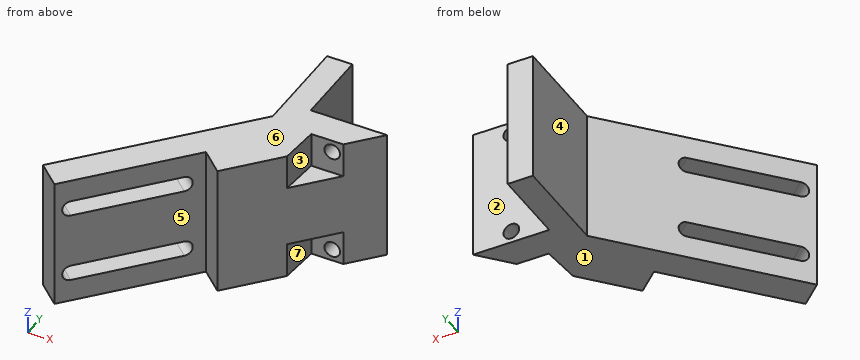
Autodesk Inventor part; units mm, degrees
ref_plane "Work Plane2" through (-4.445, -9.144, -33.02) normal (0, 0, -1) x (0, 1, 0)
ref_plane "YZ Plane" through (0, 0, 0) normal (1, 0, 0) x (0, 1, 0)
ref_plane "XZ Plane" through (0, 0, 0) normal (0, 1, 0) x (-1, 0, 0)
ref_plane "Work Plane1" through (0, 0, 0) normal (0, 0, 1) x (1, 0, 0)
sketch "Sketch1" plane through (0, 0, 0) normal (0, 0, 1) x (1, 0, 0)
  line L0 (4.129202, -9.5377) -> (6.406797, -9.5377) construction
  line L1 (9.525, -8.41296) -> (9.525, -7.435497) construction
  line L2 (-6.406797, 9.5123) -> (-4.129202, 9.5123) construction
  line L3 (-9.525, 4.116502) -> (-9.525, 6.394097) construction
  line L4 (9.314549, -9.373063) -> (-73.965447, -101.864868) construction
  line L5 (9.166309, -9.5377) -> (-73.965447, -101.864868)
  line L6 (-73.965447, -101.864868) -> (-85.121243, -91.820144)
  line L7 (6.33881, 9.756536) -> (-85.121243, -91.820144) construction
  line L8 (9.166309, -9.5377) -> (-9.997679, -9.5377)
  line L9 (-9.997679, -9.5377) -> (-9.997679, 9.756536)
  line L10 (-9.997679, 9.756536) -> (-16.347679, 9.756536)
  line L11 (-16.347679, 9.756536) -> (-16.347679, -15.439362)
  line L12 (-16.347679, -15.439362) -> (-85.121243, -91.820144)
  point P0 (0, 0)
  dimension "d0" = 124.46
  dimension "d1" = 48
  dimension "d5" = 6.35
ref_plane "Work Plane2" through (-4.445, -9.144, -33.02) normal (0, 0, -1) x (0, 1, 0)
extrude "Extrusion1" add sketch "Sketch1" against normal up to surface (33.02 mm away)
sketch "Sketch2" plane through (-73.965447, -101.864868, -33.02) normal (-0.6691306, -0.7431448, 0) x (0.7431448, -0.6691306, 0)
  line L0 (0, 33.02) -> (0, 0)
  line L1 (-15.011605, 33.02) -> (-15.011605, 0)
  line L2 (0, 0) -> (-15.011605, 0)
  line L3 (-15.011605, 0) -> (-15.011605, 26.67)
  line L4 (-15.011605, 26.67) -> (0, 26.67)
  line L5 (0, 26.67) -> (0, 0)
  line L6 (-15.011605, 33.02) -> (0, 33.02)
  point P0 (-13.193862, 33.02)
  dimension "d19" = 6.35
extrude "Extrusion2" cut sketch "Sketch2" against normal blind 25.4 contours L0 L2 L1 L4
sketch "Sketch3" plane through (-73.965447, -101.864868, -6.35) normal (0, 0, -1) x (-0.7431448, 0.6691306, 0)
  line L0 (19.8882, 12.0904) -> (19.8882, 3.175) construction
  line L1 (0, 25.4) -> (15.011605, 25.4) construction
  line L2 (15.011605, 0) -> (0, 0) construction
  line L3 (0, 0) -> (19.8882, 0) construction
  line L4 (19.8882, 0) -> (19.8882, 25.4) construction
  line L5 (19.8882, 25.4) -> (0, 25.4) construction
  line L6 (0, 25.4) -> (0, 0) construction
  line L7 (15.011605, 0) -> (19.8882, 0)
  line L8 (19.8882, 0) -> (19.8882, 25.4)
  line L9 (19.8882, 25.4) -> (15.011605, 25.4)
  line L10 (15.011605, 25.4) -> (15.011605, 0)
  point P0 (13.193862, 125.192894)
extrude "Extrusion3" add sketch "Sketch3" against normal up to surface (6.35 mm away)
sketch "Sketch4" plane through (0, 0, 0) normal (0, 0, 1) x (1, 0, 0)
  line L0 (-88.74526, -88.557064) -> (-71.749342, -69.681186) construction
  line L1 (-73.965447, -101.864868) -> (9.166309, -9.5377) construction
  line L2 (-74.314967, -94.50927) -> (-67.5166, -86.958918) construction
  line L3 (-73.965447, -101.864868) -> (-56.969529, -82.988989) construction
  line L4 (-73.965447, -101.864868) -> (-88.74526, -88.557064) construction
  line L5 (-81.390199, -88.138702) -> (-74.591832, -80.588351) construction
  line L6 (-74.314967, -94.50927) -> (-67.5166, -86.958918) construction
  line L7 (-73.144662, -95.563017) -> (-66.346296, -88.012665)
  line L8 (-68.686904, -85.905171) -> (-75.485271, -93.455523)
  arc A0 (-75.485271, -93.455523) -> (-73.144662, -95.563017) centre (-74.314967, -94.50927) ccw
  arc A1 (-66.346296, -88.012665) -> (-68.686904, -85.905171) centre (-67.5166, -86.958918) ccw
  line L9 (-81.390199, -88.138702) -> (-74.591832, -80.588351) construction
  line L10 (-80.219894, -89.192449) -> (-73.421527, -81.642098)
  line L11 (-75.762136, -79.534604) -> (-82.560503, -87.084955)
  arc A2 (-82.560503, -87.084955) -> (-80.219894, -89.192449) centre (-81.390199, -88.138702) ccw
  arc A3 (-73.421527, -81.642098) -> (-75.762136, -79.534604) centre (-74.591832, -80.588351) ccw
  point P0 (0, 0)
  point P1 (-70.915783, -90.734094)
  point P2 (-77.991015, -84.363527)
  dimension "d37" = 10.16
  dimension "d38" = 5.1816
  dimension "d39" = 5.2324
  dimension "d40" = 9.52066
  dimension "d41" = 3.1496
  dimension "d42" = 3.1496
extrude "Extrusion4" cut sketch "Sketch4" against normal through all
sketch "Sketch6" plane through (-9.997679, -9.5377, 0) normal (0, 1, 0) x (1, 0, 0)
  arc A0 (9.506526, 4.79213) -> (10.740649, 4.300966) centre (9.523849, 3.039616) ccw construction
  arc A1 (9.506526, 31.732899) -> (10.740649, 31.241734) centre (9.523849, 29.980384) ccw construction
  circle A2 centre (9.523849, 29.980384) radius 1.9685
  circle A3 centre (9.523849, 3.039616) radius 1.9685
  point P0 (9.997679, 0)
  dimension "d24" = 3.937
  dimension "d25" = 3.937
extrude "Extrusion6" cut sketch "Sketch6" against normal through all
sketch "Sketch7" plane through (9.166309, -9.5377, 0) normal (0.7431448, -0.6691306, 0) x (0, 0, -1)
  line L0 (33.02, -98.838459) -> (33.02, 0) construction
  line L1 (33.02, -9.525) -> (0, -9.525) construction
  point P0 (0, 0.954435)
sketch "Sketch8" plane through (9.166309, -9.5377, -33.02) normal (0, 0, -1) x (-1, 0, 0)
  line L0 (11.608639, 0) -> (11.608639, -12.892699) construction
  line L1 (66.135838, -73.451289) -> (0, 0) construction
  line L2 (11.608639, -7.62) -> (6.861079, -7.62) construction
  line L3 (0, 0) -> (19.163987, 0) construction
  line L4 (7.671639, 0) -> (7.671639, -8.520218) construction
  line L5 (14.910639, 0) -> (14.910639, -14.251905) construction
  line L6 (6.861079, -7.62) -> (14.910639, -7.62)
  line L7 (83.131755, -92.327168) -> (0, 0)
  line L8 (15.69062, -17.426199) -> (6.861079, -7.62)
  line L9 (15.69062, -17.426199) -> (14.910639, -7.62)
  point P0 (9.166309, 9.5377)
  dimension "d28" = 7.62
  dimension "d29" = 3.302
extrude "Extrusion7" cut sketch "Sketch8" against normal blind 8.763
sketch "Sketch9" plane through (0, 0, 0) normal (0, 0, 1) x (1, 0, 0)
  line L0 (2.30523, -17.1577) -> (-5.74433, -17.1577) construction
  line L1 (-5.74433, -17.1577) -> (-6.524312, -26.963899) construction
  line L2 (2.30523, -17.1577) -> (-6.524312, -26.963899)
  line L3 (-73.965447, -101.864868) -> (9.166309, -9.5377)
  line L4 (2.30523, -17.1577) -> (-5.74433, -17.1577)
  line L5 (-5.2705, -26.963899) -> (-5.2705, -17.1577)
  point P0 (0, 0)
sketch "Sketch9 outline for Extrusion8" plane through (0, 0, 0) normal (0, 0, 1) x (1, 0, 0)
  line L0 (-6.524312, -26.963899) -> (2.30523, -17.1577)
  line L1 (-5.74433, -17.1577) -> (-6.524312, -26.963899)
  line L2 (2.30523, -17.1577) -> (-5.74433, -17.1577)
extrude "Extrusion8" cut sketch "Sketch9 outline for Extrusion8" against normal blind 8.763
sketch "Sketch10" plane through (9.166309, -9.5377, -33.02) normal (0, 0, -1) x (-1, 0, 0)
  line L0 (25.513987, -5.901662) -> (77.291634, -63.406565)
  line L1 (67.094084, -52.081038) -> (55.938287, -62.125762)
  line L2 (66.135838, -73.451289) -> (15.69062, -17.426199) construction
  line L3 (40.913229, -45.438744) -> (36.5125, -40.551239) construction
  line L4 (66.135838, -73.451289) -> (77.291634, -63.406565) construction
  point P0 (9.166309, 9.5377)
  dimension "d34" = 15.24
sketch "Sketch11" plane through (-73.965447, -101.864868, -6.35) normal (0, 0, -1) x (-0.7431448, 0.6691306, 0)
  arc A0 (3.6068, 5.2324) -> (6.7564, 5.2324) centre (5.1816, 5.2324) ccw construction
  arc A1 (6.7564, 15.3924) -> (3.6068, 15.3924) centre (5.1816, 15.3924) ccw construction
  line L0 (5.1816, 5.2324) -> (5.1816, 15.3924) construction
  arc A2 (13.127463, 5.2324) -> (16.277063, 5.2324) centre (14.702263, 5.2324) ccw construction
  arc A3 (16.277063, 15.3924) -> (13.127463, 15.3924) centre (14.702263, 15.3924) ccw construction
  line L1 (14.702263, 5.2324) -> (14.702263, 15.3924) construction
  line L2 (14.702263, 5.2324) -> (14.702263, 15.3924) construction
  line L3 (17.877263, 5.2324) -> (17.877263, 15.3924)
  line L4 (11.527263, 15.3924) -> (11.527263, 5.2324)
  arc A4 (11.527263, 5.2324) -> (17.877263, 5.2324) centre (14.702263, 5.2324) ccw
  arc A5 (17.877263, 15.3924) -> (11.527263, 15.3924) centre (14.702263, 15.3924) ccw
  line L5 (5.1816, 5.2324) -> (5.1816, 15.3924) construction
  line L6 (8.3566, 5.2324) -> (8.3566, 15.3924)
  line L7 (2.0066, 15.3924) -> (2.0066, 5.2324)
  arc A6 (2.0066, 5.2324) -> (8.3566, 5.2324) centre (5.1816, 5.2324) ccw
  arc A7 (8.3566, 15.3924) -> (2.0066, 15.3924) centre (5.1816, 15.3924) ccw
  point P0 (13.193862, 125.192894)
  point P1 (14.702263, 10.3124)
  point P2 (5.1816, 10.3124)
  dimension "d43" = 6.35
  dimension "d44" = 6.35
extrude "Extrusion9" cut sketch "Sketch11" against normal blind 3.556
split body "Split1" sketch "Sketch10" result one side removed curves L1 removed pieces at (-50.542289, -75.103577, -13.123333)
sketch "Sketch13" plane through (9.166309, -9.5377, -33.02) normal (0, 0, -1) x (-1, 0, 0)
  line L0 (55.938287, -62.125762) -> (15.69062, -17.426199)
  line L1 (55.938287, -62.125762) -> (67.094084, -52.081038)
  line L2 (55.938287, -62.125762) -> (50.414614, -55.991102)
  line L3 (50.414614, -55.991102) -> (61.570411, -45.946377)
  line L4 (61.570411, -45.946377) -> (67.094084, -52.081038)
  line L5 (67.094084, -52.081038) -> (55.938287, -62.125762)
  point P0 (9.166309, 9.5377)
  dimension "d48" = 8.255
extrude "Extrusion10" cut sketch "Sketch13" against normal through all
sketch "Sketch15" plane through (9.166309, -9.5377, 0) normal (0.7431448, -0.6691306, 0) x (0, 0, -1)
  line L0 (7.62, -71.533459) -> (7.62, -44.863459) construction
  line L1 (0, -75.343459) -> (0, -23.449264) construction
  line L2 (0, -75.343459) -> (33.02, -75.343459) construction
  line L3 (25.4, -71.533459) -> (25.4, -44.863459) construction
  line L4 (33.02, -75.343459) -> (33.02, -23.449264) construction
  line L5 (7.62, -71.533459) -> (7.62, -44.863459) construction
  line L6 (9.5885, -71.533459) -> (9.5885, -44.863459)
  line L7 (5.6515, -44.863459) -> (5.6515, -71.533459)
  arc A0 (5.6515, -71.533459) -> (9.5885, -71.533459) centre (7.62, -71.533459) ccw
  arc A1 (9.5885, -44.863459) -> (5.6515, -44.863459) centre (7.62, -44.863459) ccw
  line L8 (25.4, -71.533459) -> (25.4, -44.863459) construction
  line L9 (27.3685, -71.533459) -> (27.3685, -44.863459)
  line L10 (23.4315, -44.863459) -> (23.4315, -71.533459)
  arc A2 (23.4315, -71.533459) -> (27.3685, -71.533459) centre (25.4, -71.533459) ccw
  arc A3 (27.3685, -44.863459) -> (23.4315, -44.863459) centre (25.4, -44.863459) ccw
  point P0 (0, 0.954435)
  point P1 (7.62, -58.198459)
  point P2 (25.4, -58.198459)
  dimension "d51" = 7.62
  dimension "d52" = 3.81
  dimension "d53" = 7.62
  dimension "d54" = 30.48
  dimension "d55" = 3.81
  dimension "d56" = 30.48
  dimension "d57" = 3.937
  dimension "d58" = 3.937
extrude "Extrusion11" cut sketch "Sketch15" against normal through all
sketch "Sketch16" plane through (9.166309, -9.5377, -33.02) normal (0, 0, -1) x (-1, 0, 0)
  line L0 (50.414614, -55.991102) -> (15.69062, -17.426199)
  line L1 (50.414614, -55.991102) -> (26.62033, -29.564872)
  line L2 (26.62033, -29.564872) -> (32.198152, -24.542578)
  line L3 (32.198152, -24.542578) -> (55.992436, -50.968808)
  line L4 (55.992436, -50.968808) -> (50.414614, -55.991102)
  point P0 (9.166309, 9.5377)
  dimension "d61" = 35.56
  dimension "d62" = 7.5057
extrude "Extrusion12" cut sketch "Sketch16" against normal through all
properties part number "arm stop 48 degree bottom half"
CAD build for the part. Positions are in the model's coordinates, mm. Face numbers are marked on the shaded views. A direction names the side the tool comes from. Round coordinates to 2 decimals unless told otherwise and drop trailing zeros. Loops run counter-clockwise (first coordinate to the right, second up) from the corner with the lowest first, then second, coordinate; pieces in that order, holes last. Notation, with made-up numbers: M 81,61.5 L 85,61.5 A23 cw 85,85.5 Z; hole C -25,87.25 d8. An arc over 180 degrees is marked long. Return JSON: item names as keys, results as strings. Group by question number.
(1) Mould opens along X. For the marked faces 4, 5, 6 and 7 say: +X half, -X half, draft (parallel to the pull), parting line (faces both ways), or undercut.
(2) Drop flat-ended pins along their axis: P1, Ø9.5, axis at y = 1, z = -20.5, coming from the +X side; P2, Ø1.5, axis at y = -47.5, z = -23, coming from the -X side; P3, Ø4.5, axis at x = -0.47, z = -29.98, coming from the -Y side. Give the stop position or say it passes through.
(3) Tool access for the marked faces 1, 2 and 3: list every direction of +Z, -Z, +X, -X, +Y, -Y with a clear straight run to the whole face (end or side of a thin tool).
(4) Saw through at C-C, the plane x = -34. List the corners of the cut face in (y, z).
(5) Saw through at A-A, the plane y = -42. List the corners of the cut face in (x, z).
(6) Wall check: probe 1 along Z at (x, y) = (-43, -50); probe 2 along Y at (x, z) = (-11, -5.5); probe 3 along Y at (x, z) = (-0.5, -6). Give the ranges that are in metal, low to high. Write a range as [from, to].
(7) Saw through at D-D, the plane z = -16.5. List the corners of the cut face in (x, y), and give its area (3 significant figures).
(8) Saw through at B-B, the plane z = -7. List the corners of the cut face in (x, y).
Answer list:
{
 "1": {"face 4": "-X half", "face 5": "undercut", "face 6": "draft", "face 7": "+X half"},
 "2": {"P1": "x = -10", "P2": "x = -45.89", "P3": "y = -17.16"},
 "3": {"face 1": "-Z, +X, -X, +Y, -Y", "face 2": "+Z, -Z, +X, +Y", "face 3": "+Z, +X, -Y"},
 "4": {"outline": "M -46.26,-33.02 L -35.04,-33.02 L -35.04,-27.37 L -46.26,-27.37 Z; M -46.26,-23.43 L -35.04,-23.43 L -35.04,-9.59 L -46.26,-9.59 Z; M -46.26,-5.65 L -35.04,-5.65 L -35.04,0 L -46.26,0 Z"},
 "5": {"outline": "M -40.26,-33.02 L -30.16,-33.02 L -30.16,-27.37 L -40.26,-27.37 Z; M -40.26,-23.43 L -30.16,-23.43 L -30.16,-9.59 L -40.26,-9.59 Z; M -40.26,-5.65 L -30.16,-5.65 L -30.16,0 L -40.26,0 Z"},
 "6": {"probe 1": "[-33.02, -27.37], [-23.43, -9.59], [-5.65, 0]", "probe 2": "[-31.93, 9.76]", "probe 3": "[-17.16, -9.54]"},
 "7": {"outline": "M -52.4,-55.48 L -46.83,-60.51 L -23.03,-34.08 L -17.45,-39.1 L 9.17,-9.54 L -10,-9.54 L -10,9.76 L -16.35,9.76 L -16.35,-15.44 Z", "area": "901 mm2"},
 "8": {"outline": "M -52.4,-55.48 L -46.83,-60.51 L -45.53,-59.06 L -51.1,-54.04 Z; M -30.76,-31.44 L -25.18,-36.47 L -23.03,-34.08 L -17.45,-39.1 L -6.52,-26.96 L -5.74,-17.16 L 2.31,-17.16 L 9.17,-9.54 L -10,-9.54 L -10,9.76 L -16.35,9.76 L -16.35,-15.44 Z"}
}
